Could you check a few things on this model? Use its own coordinates, in mm. A direction names the side the tool comes from. Coordinates: 2 decimals unless noted, no trailing zeros. Order: outer loops, then holes, each group sorted by start corner. A loop starts at its lowest first (then second) coordinate and runs counter-clockwise, first axis right, second up. Notation, with made-up numbers: (34, 7.25) - (56, 7.25) arc R34 cw to (56, 37.25) - close; hole circle Ø11 at (58.5, 17.5). An arc over 180 degrees is marked (long way). Answer as a JSON object with one key per item and string values. Group by question number.
(1) Will these pins go through, and if not, where does the flat tip stop? P1, Ø0.6, axis at x = 16, z = 51.5, coming from the +Y side; P2, Ø14, axis at x = -44.5, y = 31, coming from the +Z side; P3, Ø2, axis at y = -4.5, z = 50.5, coming from the +X side.
(2) Imagine slicing it at A-A, the plane x = 7. Write out the boundary of the cut face in (y, z), and give its area (3 significant figures).
(3) Imagine slicing it at C-C, the plane z = 6.5. Write out the boundary of the cut face in (x, y), and give its area (3 significant figures).
(4) Please list where these lines run through material, in increasing order: probe 1 along Z at (x, y) = (-32.5, -11.5); probe 2 along Y at (x, z) = (-0.5, -7); probe 3 along Y at (x, z) = (-7.5, 22).
(5) Which directions (+Z, -Z, +X, -X, +Y, -Y) give clear straight access to the entire face, cutting with the end or side of a thin tool? Please do faces 1 (the flat face through (52, -25, -15)), 2 (the flat face through (52, 28, -5)).
(6) We'd pull the mould along X, two halves only. Please class faces 3 (the flat face through (16, 12, 50)), 4 (the cylindrical face through (49.4, 45.09, -7.54)), 5 (the cylindrical face through (-40.48, -0.07, 30.49)): pulls with the +X half, pulls with the -X half, needs draft (parallel to the pull), parting line crosses it, or undercut.
from build123d import *

# Parameters (mm, degrees)
F0_W          = 150
F0_H          = 35
F1_DEPTH      = 10
F3_R          = 20
F4_DEPTH      = 5
F5_R          = 15
F6_SIZE       = 15
F7_R          = 4.99999
F10_DEPTH     = 40
F11_DEPTH     = 25
F12_R         = 15
F14_W         = 3
F14_H         = 40
F15_DEPTH     = 2
F16_T3_ANGLE  = 273.8677552215
F16_T7_ANGLE  = 273.8677552215
F16_T11_ANGLE = 245.1581434466
F16_T15_ANGLE = 245.1581434466


# Not quite as in the source:
# - a fillet or chamfer that OpenCascade refuses, or shapes differently, is made with other operations: its cross-section is extruded or revolved along the edge and cut away or added
# - a fillet or chamfer is up to 0.001 mm smaller than in the source, because OpenCascade refuses the exact size


with BuildPart() as f1:
    # F0 (on Top) → F1 (new body, symmetric)
    with BuildSketch(Plane.XY):
        Rectangle(F0_W, F0_H)
    extrude(amount=F1_DEPTH, both=True)

    # F3 (on offset) → F4 (join, symmetric)
    with BuildSketch(Plane.XY.offset(-10)):
        with Locations((-52, -25.2603590488)):
            Circle(F3_R)
        with Locations((52, -25.2603590488)):
            Circle(F3_R)
        with Locations((52, 25.2603590488)):
            Circle(F3_R)
        with Locations((-52, 25.2603590488)):
            Circle(F3_R)
    extrude(amount=F4_DEPTH, both=True)

    # F5
    f5_edges = [f1.edges().sort_by_distance(p)[0] for p in [
        (-75, 0, 10),
    ]]
    fillet(f5_edges, radius=F5_R)

    # F6
    f6_edges = [f1.edges().sort_by_distance(p)[0] for p in [
        (75, 0, 10),
    ]]
    chamfer(f6_edges, length=F6_SIZE)

    # F7 (radius 5 in the source; OpenCascade refuses exactly that, so slightly less here)
    f7_edges = [f1.edges().sort_by_distance(p)[0] for p in [
        (32, -25.260359, -15),
        (32, 25.260359, -15),
        (-72, -25.260359, -15),
        (-72, 25.260359, -15),
    ]]
    fillet(f7_edges, radius=F7_R)

    # F9 (on offset) → F10 (join)
    with BuildSketch(Plane.XY.offset(10)):
        with BuildLine():
            ThreePointArc((15.0216268376, 5), (10.0216268376, 0), (15.0216268376, -5))
            ThreePointArc((15.0216268376, -5), (18.5571607435, -3.5355339059), (20.0216268376, 0))
            ThreePointArc((20.0216268376, 0), (18.5571607435, 3.5355339059), (15.0216268376, 5))
        make_face()
    extrude(amount=F10_DEPTH)

    # F9 (on offset) → F11 (join)
    with BuildSketch(Plane.XY.offset(10)):
        with BuildLine():
            Line((-44.7599912546, -5), (15.0216268376, -5))
            ThreePointArc((15.0216268376, -5), (10.0216268376, 0), (15.0216268376, 5))
            Line((15.0216268376, 5), (-44.7599912546, 5))
            Line((-44.7599912546, 5), (-44.7599912546, -5))
        make_face()
    extrude(amount=F11_DEPTH)

    # F12
    f12_edges = [f1.edges().sort_by_distance(p)[0] for p in [
        (-44.759991, 0, 35),
    ]]
    fillet(f12_edges, radius=F12_R)

    # F14 (on offset) → F15 (join)
    with BuildSketch(Plane.XY.offset(50)):
        with Locations((15.6161214935, 0)):
            Rectangle(F14_W, F14_H)
    extrude(amount=F15_DEPTH)

    # F16: fillet of radius 2 on 2 edges, made by hand


with BuildPart() as f16_tool1:
    # F16_s2 → F16_t3 (revolve)
    with BuildSketch(Plane(origin=(7.0041804705, 7.4937067775, 0), x_dir=(0, 0, 1), z_dir=(0.6828419269, 0.7305661522, 0))):
        with BuildLine():
            ThreePointArc((48, 15.9742921192), (49.4142135624, 15.3885056815), (50, 13.9742921192))
            Line((50, 13.9742921192), (50, 15.9742921192))
            Line((50, 15.9742921192), (48, 15.9742921192))
        make_face()
    revolve(axis=Axis((15.0216268376, 0, 50), (0, 0, -1)), revolution_arc=F16_T3_ANGLE)

    split(bisect_by=Plane.YZ.offset(17.1161214935), keep=Keep.TOP)


with BuildPart() as f16_tool5:
    # F16_s6 → F16_t7 (revolve)
    with BuildSketch(Plane(origin=(7.0041804705, 7.4937067775, 0), x_dir=(0, 0, 1), z_dir=(0.6828419269, 0.7305661522, 0))):
        with BuildLine():
            ThreePointArc((48, 15.9742921192), (49.4142135624, 15.3885056815), (50, 13.9742921192))
            Line((50, 13.9742921192), (50, 15.9742921192))
            Line((50, 15.9742921192), (48, 15.9742921192))
        make_face()
    revolve(axis=Axis((15.0216268376, 0, 50), (0, 0, -1)), revolution_arc=F16_T7_ANGLE)

    split(bisect_by=Plane.YZ.offset(14.1161214935), keep=Keep.BOTTOM)


with BuildPart() as f16_tool9:
    # F16_s10 → F16_t11 (revolve)
    with BuildSketch(Plane(origin=(10.6662198, 6.8158439522, 0), x_dir=(0, 0, 1), z_dir=(-0.8426491362, -0.5384630287, 0))):
        with BuildLine():
            ThreePointArc((48, -3.0885906834), (49.4142135624, -3.674377121), (50, -5.0885906834))
            Line((50, -5.0885906834), (50, -3.0885906834))
            Line((50, -3.0885906834), (48, -3.0885906834))
        make_face()
    revolve(axis=Axis((15.0216268376, 0, 50), (0, 0, -1)), revolution_arc=F16_T11_ANGLE)

    split(bisect_by=Plane.YZ.offset(14.1161214935), keep=Keep.BOTTOM)


with BuildPart() as f16_tool13:
    # F16_s14 → F16_t15 (revolve)
    with BuildSketch(Plane(origin=(10.6662198, 6.8158439522, 0), x_dir=(0, 0, 1), z_dir=(-0.8426491362, -0.5384630287, 0))):
        with BuildLine():
            ThreePointArc((48, -3.0885906834), (49.4142135624, -3.674377121), (50, -5.0885906834))
            Line((50, -5.0885906834), (50, -3.0885906834))
            Line((50, -3.0885906834), (48, -3.0885906834))
        make_face()
    revolve(axis=Axis((15.0216268376, 0, 50), (0, 0, -1)), revolution_arc=F16_T15_ANGLE)

    split(bisect_by=Plane.YZ.offset(17.1161214935), keep=Keep.TOP)


with BuildPart() as f1_1:
    add(f1.part)

    # F16_t17: cut F16_tool1, F16_tool5, F16_tool9, F16_tool13
    add([f16_tool1.part, f16_tool5.part, f16_tool9.part, f16_tool13.part], mode=Mode.SUBTRACT)


solid = f1_1.part
Result set:
{
 "1": {"P1": "stops at y = 20", "P2": "stops at z = -5", "P3": "stops at x = 17.12"},
 "2": {"outline": "(-17.5, -10) - (17.5, -10) - (17.5, 10) - (5, 10) - (5, 35) - (-5, 35) - (-5, 10) - (-17.5, 10) - close", "area": "950 mm^2"},
 "3": {"outline": "(-69.63, -17.5) - (63.5, -17.5) - (63.5, 17.5) - (-69.63, 17.5) - close", "area": "4,660 mm^2"},
 "4": {"probe 1": "z = -10 to 10", "probe 2": "y = -17.5 to 17.5", "probe 3": "y = -5 to 5"},
 "5": {"face 1": "-Z, +X, -X, +Y, -Y", "face 2": "+Z, +X, -X, +Y"},
 "6": {"face 3": "needs draft", "face 4": "undercut", "face 5": "pulls with the -X half"}
}
